```python
from build123d import *

# Parameters (mm, degrees)
SKETCH_3_R          = 2.25
CUT_EXTRUDE_1_DEPTH = 10
SKETCH_4_R          = 5
CUT_EXTRUDE_2_DEPTH = 6


with BuildPart() as part:
    # Эскиз2 → Повернуть1 (revolve)
    with BuildSketch(Plane.XY, mode=Mode.PRIVATE) as revolve_1_sk:
        Polygon((0, 4.367021277), (-7.5, 4.367021277), (-11, -5.632978723), (0, -5.632978723), align=None)
    revolve(revolve_1_sk.sketch.rotate(Axis((0, -5.632978723, 0), (0, 1, 0)), 270), axis=Axis((0, -5.632978723, 0), (0, 1, 0)))

    # Эскиз3 → Вырез-Вытянуть1 (cut)
    with BuildSketch(Plane(origin=(0, 4.367021277, 0), x_dir=(1, 0, 0), z_dir=(0, 1, 0))):
        with Locations(Location((0, 0, 0), (0, 0, 270))):
            Circle(SKETCH_3_R)
    extrude(amount=-CUT_EXTRUDE_1_DEPTH, mode=Mode.SUBTRACT)

    # Эскиз4 → Вырез-Вытянуть2 (cut)
    with BuildSketch(Plane(origin=(0, 4.367021277, 0), x_dir=(1, 0, 0), z_dir=(0, 1, 0))):
        with Locations(Location((0, 0, 0), (0, 0, 270))):
            Circle(SKETCH_4_R)
    extrude(amount=-CUT_EXTRUDE_2_DEPTH, mode=Mode.SUBTRACT)


solid = part.part
```
Geometry: final body of the model. Coordinates: model frame, mm. A direction names the side the tool comes from. Coordinates: 2 decimals unless noted, no trailing zeros. Order: outer loops, then holes, each group sorted by start corner. A loop starts at its lowest first (then second) coordinate and runs counter-clockwise, first axis right, second up. Notation, with made-up numbers: (83, 22.5) -> (100, 22.5) arc R36 ccw to (100, 61.5) -> close; hole circle Ø11 at (12.25, 37). An arc over 180 degrees is marked (long way). Write each question's results on one line, items separated by ' | '. Start each with the question number.
1) Cut plane B-B, the plane z = 0. Output: boundary loops of the cut face in (x, y).
2) Cut plane A-A, the plane x = 0. Output: boundary loops of the cut face in (y, z).
3) Cut plane C-C, the plane y = 0.75. Output: boundary loops of the cut face in (x, z).
4) First-contact query: pin 1 (2 mm diameter, centred on x = 4.5, y = 1.5, fed in from -Z); pin 2 (6 mm diameter, centred on x = -8, z = 3.5, fed in from +Y); pin 3 (2.5 mm diameter, centred on x = 0, z = 0, fed in from +Y); pin 4 (5 mm diameter, centred on x = 7.5, y = 1, fed in from +Z). Flat tips, straight axial feed; report the tip coordinate or a pass-through.
5) Material intervals for line 1 along Y through (x, z) = (-1, -3); line 2 along X through (y, z) = (1.4, 0); line 3 along Z through (x, y) = (-4.5, 1), sorted ascending.
6) Mould query, pull axis Y, two halves, no side actions, for faces 3 (the cylindrical face through (0.676, -3.605, 2.146)), 4 (the flat face through (-1, -1.633, 2.2)), 5 (the flat face through (-3, -5.633, 0)). Classes: released by +Y, released by -Y, zero draft, split by the parting line, or undercut.
7) Set-up query: faces 1 (the cylindrical face through (-4.88, 1.41, -1.08)), 2 (the flat face through (2, 4.367, 5)). Return all of +Z, -Z, +X, -X, +Y, -Y with unobstructed straight access to the full face (end or side cutting, diameter ignored); none if empty.
Checks:
1) outline: (-11, -5.63) -> (-2.25, -5.63) -> (-2.25, -1.63) -> (-5, -1.63) -> (-5, 4.37) -> (-7.5, 4.37) -> close; (2.25, -5.63) -> (11, -5.63) -> (7.5, 4.37) -> (5, 4.37) -> (5, -1.63) -> (2.25, -1.63) -> close
2) outline: (-5.63, -11) -> (4.37, -7.5) -> (4.37, -5) -> (-1.63, -5) -> (-1.63, -2.25) -> (-5.63, -2.25) -> close; (-5.63, 2.25) -> (-1.63, 2.25) -> (-1.63, 5) -> (4.37, 5) -> (4.37, 7.5) -> (-5.63, 11) -> close
3) outline: circle Ø17.53 at (0, 0); hole circle Ø10 at (0, 0)
4) pin 1: z = -7.89 | pin 2: y = 4.37 | pin 3: through | pin 4: z = 7.39
5) line 1: -5.63 to -1.63 | line 2: -8.54 to -5, 5 to 8.54 | line 3: -7.42 to -2.18, 2.18 to 7.42
6) face 3: zero draft | face 4: released by +Y | face 5: released by -Y
7) face 1: +Y | face 2: +Z, -Z, +X, -X, +Y
